```python
from build123d import *

# Parameters (mm, degrees)
BOSS_EXTRUDE1_DEPTH = 11
SKETCH2_R           = 3
CUT_EXTRUDE1_DEPTH  = 30
CUT_EXTRUDE3_DEPTH  = 9
FILLET2_R           = 2.36
FILLET3_R           = 2.36


with BuildPart() as part:
    # Sketch1 → Boss-Extrude1 (new body)
    with BuildSketch(Plane(origin=(0, 0, 0), x_dir=(1, 0, 0), z_dir=(0, 1, 0))):
        with BuildLine():
            Line((-27.916231576, -22.71939994), (27.916231576, -22.71939994))
            Line((27.916231576, -22.71939994), (27.916231576, -3.602655093))
            Line((27.916231576, -3.602655093), (13.916231576, -3.602655093))
            ThreePointArc((13.916231576, -3.602655093), (0, -14.375), (-13.916231576, -3.602655093))
            Line((-13.916231576, -3.602655093), (-27.916231576, -3.602655093))
            Line((-27.916231576, -3.602655093), (-27.916231576, -22.71939994))
        make_face()
    extrude(amount=BOSS_EXTRUDE1_DEPTH)

    # Sketch2 → Cut-Extrude1 (cut)
    with BuildSketch(Plane(origin=(0, 0, 3.602655093), x_dir=(-1, 0, 0), z_dir=(0, 0, -1))):
        with Locations((22.416231576, 5.5)):
            Circle(SKETCH2_R)
        with Locations((-22.416231576, 5.5)):
            Circle(SKETCH2_R)
    extrude(amount=-CUT_EXTRUDE1_DEPTH, mode=Mode.SUBTRACT)

    # Sketch3 → Cut-Extrude3 (cut)
    with BuildSketch(Plane(origin=(0, 11, 0), x_dir=(1, 0, 0), z_dir=(0, 1, 0))):
        with BuildLine():
            Line((-17.288574276, -6.224614407), (-17.288574276, -22.71939994))
            Line((-17.288574276, -22.71939994), (-3, -22.71939994))
            Line((-3, -22.71939994), (-3, -18.128447948))
            ThreePointArc((-3, -18.128447948), (-11.761457171, -14.1176751), (-17.288574276, -6.224614407))
        make_face()
        with BuildLine():
            Line((3, -18.128447948), (3, -22.71939994))
            Line((3, -22.71939994), (17.288574276, -22.71939994))
            Line((17.288574276, -22.71939994), (17.288574276, -6.224614407))
            ThreePointArc((17.288574276, -6.224614407), (11.761457171, -14.1176751), (3, -18.128447948))
        make_face()
    extrude(amount=-CUT_EXTRUDE3_DEPTH, mode=Mode.SUBTRACT)

    # Fillet2
    fillet2_edges = [part.edges().sort_by_distance(p)[0] for p in [
        (-17.288574276, 6.5, 6.224614407),
        (-3, 6.5, 18.128447948),
        (3, 6.5, 18.128447948),
        (17.288574276, 6.5, 6.224614407),
    ]]
    fillet(fillet2_edges, radius=FILLET2_R)

    # Fillet3
    fillet3_edges = [part.edges().sort_by_distance(p)[0] for p in [
        (27.916231576, 11, 13.161027516),
        (-27.916231576, 11, 13.161027516),
        (27.916231576, 0, 13.161027516),
        (-27.916231576, 0, 13.161027516),
    ]]
    fillet(fillet3_edges, radius=FILLET3_R)


solid = part.part
```
Source: CAD feature listing. Evaluate the final solid. Frame: model axes, mm. A direction names the side the tool comes from. Give positions to 0.01 mm unless a question says otherwise; leave off trailing zeros. Loops run counter-clockwise (first coordinate to the right, second up) from the corner with the lowest first, then second, coordinate; pieces in that order, holes last. Notation, with made-up numbers: (-12.5, 70) - (13.5, 70) arc R36 cw to (13.5, 104) - close; hole circle Ø5 at (-28.75, 42.5). An arc over 180 degrees is marked (long way). Use CSV: the item, a comma, the result in double quotes. Start each with the question number.
1. Section B-B (z = 13.5). Output: boundary loops of the cut face in (x, y), then the cut area to 4 significant figures.
2. Draft query along Y for faces 1 (the cylindrical face through (-27.243, 0.71, 13.295)), 2 (the cylindrical face through (-15.848, 6.437, 12.217)), 3 (the cylindrical face through (19.645, 4.351, 13.027)), 4 (the cylindrical face through (-19.42, 5.63, 13.03)). Return one class per face: +Y half, -Y half, draft (parallel to the pull), parting line (faces both ways), or undercut.
3. Section C-C (x = -22). Output: boundary loops of the cut face in (y, z), then the cut area to 3 significant figures.
4. Ray query, L1, parallel to X at y = 6, z = 20.25; L2, parallel to X at y = 4.5, z = 16; L3, parallel to X at y = 9.25, z = 15.25. Return the intervals inside material, ascending.
5. Section A-A (y = 5.5). Output: boundary loops of the cut face in (x, z) (3 decimals).
6. Reachability of faces 5 (the cylindrical face through (15.848, 6.437, 12.217)), 6 (the flat face through (27.916, 5, 13)) from +Z, -Z, +X, -X, +Y, -Y: full face, straight path, thin tool, end or side. Return the list, or none.
7. Section D-D (z = 10.25). Output: boundary loops of the cut face in (x, y).
8. Pin query (flat end, axial travel): pin 1 (5.5 mm diameter, centred on x = 9.5, z = 19.5, fed in from +Y); pin 2 (5.5 mm diameter, centred on x = -22.42, y = 5.5, fed in from +Z). Return the tip coordinate at first contact, or that it passes through.
Response:
1,outline,"(-27.92, 2.36) arc R2.36 ccw to (-25.56, 0) - (-4.94, 0) - (-4.94, 11) - (-12.47, 11) - (-12.47, 2) - (-17.11, 2) - (-17.11, 11) - (-25.56, 11) arc R2.36 ccw to (-27.92, 8.64) - close; (4.94, 0) - (25.56, 0) arc R2.36 ccw to (27.92, 2.36) - (27.92, 8.64) arc R2.36 ccw to (25.56, 11) - (17.11, 11) - (17.11, 2) - (12.47, 2) - (12.47, 11) - (4.94, 11) - close; hole circle Ø6 at (-22.42, 5.5); hole circle Ø6 at (22.42, 5.5)"
1,area,"360.5 mm²"
2,face 1,"-Y half"
2,face 2,"draft"
2,face 3,"undercut"
2,face 4,"undercut"
3,outline,"(0, 3.6) - (2.53, 3.6) - (2.53, 22.72) - (0, 22.72) - close; (8.47, 3.6) - (11, 3.6) - (11, 22.72) - (8.47, 22.72) - close"
3,area,"96.7 mm²"
4,L1,"-27.92 to -25.37, -19.46 to -17.29, -3 to 3, 17.29 to 19.46, 25.37 to 27.92"
4,L2,"-27.92 to -25.24, -19.59 to -17.29, -9.04 to 9.04, 17.29 to 19.59, 25.24 to 27.92"
4,L3,"-27.84 to -17.29, -10.25 to 10.25, 17.29 to 27.84"
5,outline,"(-27.916, 3.603) - (-25.416, 3.603) - (-25.416, 22.719) - (-27.916, 22.719) - close; (-19.416, 3.603) - (-13.916, 3.603) arc R14.375 cw to (13.916, 3.603) - (19.416, 3.603) - (19.416, 22.719) - (17.289, 22.719) - (17.289, 14.39) arc R2.36 cw to (13.229, 12.752) arc R18.375 ccw to (4.75, 17.75) arc R2.36 cw to (3, 20.03) - (3, 22.719) - (-3, 22.719) - (-3, 20.03) arc R2.36 cw to (-4.75, 17.75) arc R18.375 ccw to (-13.229, 12.752) arc R2.36 cw to (-17.289, 14.39) - (-17.289, 22.719) - (-19.416, 22.719) - close; (25.416, 3.603) - (27.916, 3.603) - (27.916, 22.719) - (25.416, 22.719) - close"
6,face 5,"+Z, +Y"
6,face 6,"+Z, -Z, +X, +Y, -Y"
7,outline,"(-27.92, 2.36) arc R2.36 ccw to (-25.56, 0) - (-10.08, 0) - (-10.08, 11) - (-25.56, 11) arc R2.36 ccw to (-27.92, 8.64) - close; (10.08, 0) - (25.56, 0) arc R2.36 ccw to (27.92, 2.36) - (27.92, 8.64) arc R2.36 ccw to (25.56, 11) - (10.08, 11) - close; hole circle Ø6 at (-22.42, 5.5); hole circle Ø6 at (22.42, 5.5)"
8,pin 1,"y = 2"
8,pin 2,"through"
